Source: CAD feature listing. Evaluate the final solid. Frame: model axes, mm. Give positions to 0.01 mm unless a question says otherwise; leave off trailing zeros. Write each loop counter-clockwise with the first axis right and the second up, starting at its lowest first coordinate (ties: lowest second). Pieces come first, ordered by that corner, then holes. Notation, with made-up numbers: (76.25, 70.25) - (102.25, 70.25) arc R25 cw to (102.25, 109.25) - close; hole circle Ø5 at (14.25, 9.5). An arc over 180 degrees is marked (long way). One line per question, with ' | ' between items. Start each with the question number.
(1) Pin query (flat end, axial travel): pin 1 (2.5 mm diameter, centred on x = 28, y = 27.5, fed in from +Z); pin 2 (3 mm diameter, centred on x = -15.5, z = 2.5, fed in from -Y); pin 3 (1.5 mm diameter, centred on x = 22, z = 5.5, fed in from -Y). Return the tip coordinate at first contact, or that it passes through.
(2) Section B-B, the plane x = 5.5. Return loops of the section in (y, z), plus the area to 3 significant figures.
(3) Section A-A, the plane y = -10. Return loops of the section in (x, z).
(4) Ray query, line 1 (X direction, y = 1, z = 2.5); line 2 (X direction, y = 22, z = 4); line 3 (Y direction, x = -32.5, z = 4.25). Return the intervals inside material, ascending. Write a range as [from, to].
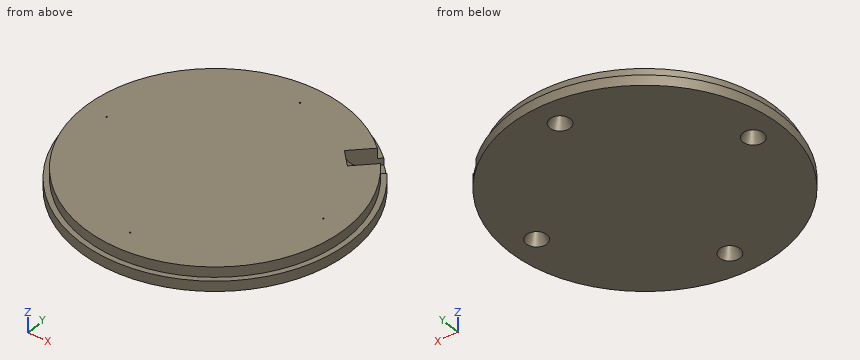
Autodesk Fusion 360 part; units mm, degrees
sketch "Sketch1" plane through (0, 0, 0) normal (0, 0, 1) x (1, 0, 0)
  circle A0 centre (0, 0) radius 40
  dimension "d1" = 80
extrude "Extrude1" add sketch "Sketch1" along normal blind 3
sketch "Sketch2" plane through (0, 0, 3) normal (0, 0, 1) x (-1, 0, 0)
  circle A0 centre (0, 0) radius 40
  circle A1 centre (0, 0) radius 38.5
  circle A2 centre (0, 32) radius 3.75
  circle A3 centre (0, 32) radius 5.5
  circle A4 centre (0, 0) radius 37
  dimension "d4" = 77
  dimension "d5" = 7.5
  dimension "d6" = 11
  dimension "d7" = 32
  dimension "d8" = 74
extrude "Extrude2" add sketch "Sketch2" along normal blind 3 contours A1 | A3 A4 | A3 A4 picked at (-1.5513, 36.4665) picked at (-0.1427, -15.7625)
pattern_circular "C-Pattern1" count 4 over 360 about axis through (0, 0, 1.75) along (0, 0, 1) of "Extrude2"
sketch "Sketch3" plane through (0, 0, 0) normal (0, 0, -1) x (1, 0, 0)
  circle A0 centre (0, 0) radius 40
  circle A1 centre (0, -32) radius 3
  dimension "d13" = 6
  dimension "d14" = 32
extrude "Extrude3" cut sketch "Sketch3" against normal through all draft -25 contours A1
pattern_circular "C-Pattern2" count 4 over 360 about axis through (0, 0, 0) along (0, 0, 1) of "Extrude3"
ref_plane "WorkPlane1" through (0, 0, 0) normal (-0.7071, 0.7071, 0) x (0, 0, 1)
sketch "Sketch4" plane through (0, 0, 0) normal (-0.7071, 0.7071, 0) x (0, 0, 1)
  line L0 (6, -27.2236) -> (6, 38.5)
  line L1 (6, -38.5) -> (6, -27.2236)
  line L2 (3, -40) -> (3, -38.5)
  line L3 (3, 38.5) -> (3, 40)
  line L4 (0, -40) -> (0, 40)
  line L5 (3, -38.5) -> (6, -38.5)
  line L6 (3, 38.5) -> (6, 38.5)
  line L7 (0, -40) -> (3, -40)
  line L8 (0, 40) -> (3, 40)
  line L9 (3, 40) -> (6, 40)
  line L10 (6, 40) -> (6, 30.653)
  line L11 (3, 40) -> (1, 40)
  line L12 (1, 40) -> (1, 35.115)
  arc A0 (1, 35.115) -> (6, 30.653) centre (5.4909, 35.115) ccw
  dimension "d18" = 3
  dimension "d19" = 9.347
  dimension "d20" = 2
  dimension "d21" = 4.885
extrude "Extrude4" cut sketch "Sketch4" along normal mid plane 6 contours L0 L3 L6 L8 L10 L11 L12 A0 | L3 L6 L9 L10
Check sheet entries:
1) pin 1: z = 1 | pin 2: y = -37.47 | pin 3: y = -32.1
2) outline: (-39.62, 0) - (39.62, 0) - (39.62, 3) - (38.11, 3) - (38.11, 6) - (-38.11, 6) - (-38.11, 3) - (-39.62, 3) - close | area: 466 mm²
3) outline: (-38.73, 0) - (38.73, 0) - (38.73, 3) - (37.18, 3) - (37.18, 6) - (-37.18, 6) - (-37.18, 3) - (-38.73, 3) - close
4) line 1: [-39.99, -33.54], [-30.46, 30.46], [33.54, 39.99] | line 2: [-31.6, 21.67], [26.24, 31.6] | line 3: [-20.64, -0.89], [0.89, 20.64]
